from build123d import *

# Parameters (mm, degrees)
BOSS_EXTRUDE1_DEPTH = 4
CUT_EXTRUDE1_REACH  = 6
SKETCH2_R           = 11.5
SKETCH2_R_2         = 1.6
CUT_EXTRUDE2_REACH  = 6
SKETCH4_R           = 1.5
SKETCH5_W           = 10
SKETCH5_H           = 30
BOSS_EXTRUDE2_DEPTH = 12
FILLET1_R           = 1.5
CUT_EXTRUDE3_REACH  = 6
SKETCH6_R           = 4


with BuildPart() as part:
    # Sketch1 → Boss-Extrude1 (new body)
    with BuildSketch(Plane.XZ.offset(-57.396189287)):
        with BuildLine():
            Line((117.077991716, 202.076411562), (117.077991716, 81.069101486))
            add(Edge.make_bspline(
                [(111.081646754, 75.072756524), (117.077991716, 75.072756524), (117.077991716, 81.069101486)],
                knots=[5.498396131, 5.498396131, 5.498396131, 7.067974483, 7.067974483, 7.067974483], degree=2, weights=[1, 0.707537269, 1]))
            Line((111.081646754, 75.072756524), (4.474336679, 75.072756524))
            add(Edge.make_bspline(
                [(-1.522008284, 81.069101486), (-1.522008284, 75.072756524), (4.474336679, 75.072756524)],
                knots=[5.498396131, 5.498396131, 5.498396131, 7.067974483, 7.067974483, 7.067974483], degree=2, weights=[1, 0.707537269, 1]))
            Line((-1.522008284, 81.069101486), (-1.522008284, 202.076411562))
            add(Edge.make_bspline(
                [(4.474336679, 208.072756524), (-1.522008284, 208.072756524), (-1.522008284, 202.076411562)],
                knots=[5.498396131, 5.498396131, 5.498396131, 7.067974483, 7.067974483, 7.067974483], degree=2, weights=[1, 0.707537269, 1]))
            Line((4.474336679, 208.072756524), (111.081646754, 208.072756524))
            add(Edge.make_bspline(
                [(117.077991716, 202.076411562), (117.077991716, 208.072756524), (111.081646754, 208.072756524)],
                knots=[5.498396131, 5.498396131, 5.498396131, 7.067974483, 7.067974483, 7.067974483], degree=2, weights=[1, 0.707537269, 1]))
        make_face()
    extrude(amount=BOSS_EXTRUDE1_DEPTH)

    # Sketch2 → Cut-Extrude1 (cut, up to next)
    with BuildSketch(Plane.XZ.offset(-53.396189287), mode=Mode.PRIVATE) as cut_extrude1_sk1:
        with Locations((57.631208462, 183.071537466)):
            Circle(SKETCH2_R)
    cut_extrude1_tool1 = extrude(cut_extrude1_sk1.sketch, amount=-CUT_EXTRUDE1_REACH, mode=Mode.PRIVATE) & part.part
    add(cut_extrude1_tool1.solids().sort_by_distance((57.631208, 53.396189, 183.071537))[0], mode=Mode.SUBTRACT)
    # Sketch2 → Cut-Extrude1 (cut, up to next)
    with BuildSketch(Plane.XZ.offset(-53.396189287), mode=Mode.PRIVATE) as cut_extrude1_sk2:
        with Locations((73.131208462, 198.571537436)):
            Circle(SKETCH2_R_2)
    cut_extrude1_tool2 = extrude(cut_extrude1_sk2.sketch, amount=-CUT_EXTRUDE1_REACH, mode=Mode.PRIVATE) & part.part
    add(cut_extrude1_tool2.solids().sort_by_distance((73.131208, 53.396189, 198.571537))[0], mode=Mode.SUBTRACT)
    # Sketch2 → Cut-Extrude1 (cut, up to next)
    with BuildSketch(Plane.XZ.offset(-53.396189287), mode=Mode.PRIVATE) as cut_extrude1_sk3:
        with Locations((42.131208462, 198.571537436)):
            Circle(SKETCH2_R_2)
    cut_extrude1_tool3 = extrude(cut_extrude1_sk3.sketch, amount=-CUT_EXTRUDE1_REACH, mode=Mode.PRIVATE) & part.part
    add(cut_extrude1_tool3.solids().sort_by_distance((42.131208, 53.396189, 198.571537))[0], mode=Mode.SUBTRACT)
    # Sketch2 → Cut-Extrude1 (cut, up to next)
    with BuildSketch(Plane.XZ.offset(-53.396189287), mode=Mode.PRIVATE) as cut_extrude1_sk4:
        with Locations((42.131208462, 167.571537436)):
            Circle(SKETCH2_R_2)
    cut_extrude1_tool4 = extrude(cut_extrude1_sk4.sketch, amount=-CUT_EXTRUDE1_REACH, mode=Mode.PRIVATE) & part.part
    add(cut_extrude1_tool4.solids().sort_by_distance((42.131208, 53.396189, 167.571537))[0], mode=Mode.SUBTRACT)
    # Sketch2 → Cut-Extrude1 (cut, up to next)
    with BuildSketch(Plane.XZ.offset(-53.396189287), mode=Mode.PRIVATE) as cut_extrude1_sk5:
        with Locations((73.131208462, 167.571537436)):
            Circle(SKETCH2_R_2)
    cut_extrude1_tool5 = extrude(cut_extrude1_sk5.sketch, amount=-CUT_EXTRUDE1_REACH, mode=Mode.PRIVATE) & part.part
    add(cut_extrude1_tool5.solids().sort_by_distance((73.131208, 53.396189, 167.571537))[0], mode=Mode.SUBTRACT)

    # Sketch4 → Cut-Extrude2 (cut, up to next)
    with BuildSketch(Plane.XZ.offset(-53.396189287), mode=Mode.PRIVATE) as cut_extrude2_sk1:
        with Locations((8.994115753, 197.556632488)):
            Circle(SKETCH4_R)
    cut_extrude2_tool1 = extrude(cut_extrude2_sk1.sketch, amount=-CUT_EXTRUDE2_REACH, mode=Mode.PRIVATE) & part.part
    add(cut_extrude2_tool1.solids().sort_by_distance((8.994116, 53.396189, 197.556632))[0], mode=Mode.SUBTRACT)
    # Sketch4 → Cut-Extrude2 (cut, up to next)
    with BuildSketch(Plane.XZ.offset(-53.396189287), mode=Mode.PRIVATE) as cut_extrude2_sk2:
        with Locations((106.56186768, 197.556632488)):
            Circle(SKETCH4_R)
    cut_extrude2_tool2 = extrude(cut_extrude2_sk2.sketch, amount=-CUT_EXTRUDE2_REACH, mode=Mode.PRIVATE) & part.part
    add(cut_extrude2_tool2.solids().sort_by_distance((106.561868, 53.396189, 197.556632))[0], mode=Mode.SUBTRACT)
    # Sketch4 → Cut-Extrude2 (cut, up to next)
    with BuildSketch(Plane.XZ.offset(-53.396189287), mode=Mode.PRIVATE) as cut_extrude2_sk3:
        with Locations((8.994115753, 85.588880561)):
            Circle(SKETCH4_R)
    cut_extrude2_tool3 = extrude(cut_extrude2_sk3.sketch, amount=-CUT_EXTRUDE2_REACH, mode=Mode.PRIVATE) & part.part
    add(cut_extrude2_tool3.solids().sort_by_distance((8.994116, 53.396189, 85.588881))[0], mode=Mode.SUBTRACT)
    # Sketch4 → Cut-Extrude2 (cut, up to next)
    with BuildSketch(Plane.XZ.offset(-53.396189287), mode=Mode.PRIVATE) as cut_extrude2_sk4:
        with Locations((106.56186768, 85.588880561)):
            Circle(SKETCH4_R)
    cut_extrude2_tool4 = extrude(cut_extrude2_sk4.sketch, amount=-CUT_EXTRUDE2_REACH, mode=Mode.PRIVATE) & part.part
    add(cut_extrude2_tool4.solids().sort_by_distance((106.561868, 53.396189, 85.588881))[0], mode=Mode.SUBTRACT)

    # Sketch5 → Boss-Extrude2 (add)
    with BuildSketch(Plane.XZ.offset(-53.396189287)):
        with Locations((57.477991716, 148.072756524)):
            Rectangle(SKETCH5_W, SKETCH5_H)
    extrude(amount=BOSS_EXTRUDE2_DEPTH)

    # Fillet1
    fillet1_edges = [part.edges().sort_by_distance(p)[0] for p in [
        (52.477991716, 53.396189287, 148.072756524),
        (52.477991716, 47.396189287, 163.072756524),
        (57.477991716, 53.396189287, 133.072756524),
        (52.477991716, 47.396189287, 133.072756524),
        (62.477991716, 53.396189287, 148.072756524),
        (62.477991716, 47.396189287, 133.072756524),
        (57.477991716, 53.396189287, 163.072756524),
        (62.477991716, 47.396189287, 163.072756524),
    ]]
    fillet(fillet1_edges, radius=FILLET1_R)

    # Sketch6 → Cut-Extrude3 (cut, up to next)
    with BuildSketch(Plane.XZ.offset(-53.396189287), mode=Mode.PRIVATE) as cut_extrude3_sk1:
        with Locations((38.477991716, 158.072756524)):
            Circle(SKETCH6_R)
    cut_extrude3_tool1 = extrude(cut_extrude3_sk1.sketch, amount=-CUT_EXTRUDE3_REACH, mode=Mode.PRIVATE) & part.part
    add(cut_extrude3_tool1.solids().sort_by_distance((38.477992, 53.396189, 158.072757))[0], mode=Mode.SUBTRACT)


solid = part.part
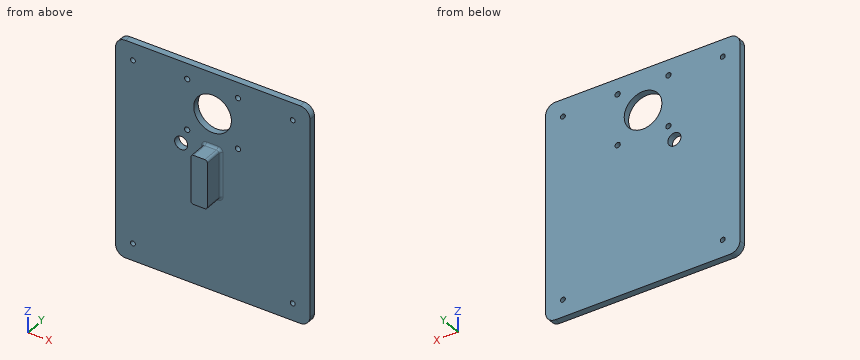
Model file for the job. Use its own axes, mm. Give positions to 0.01 mm unless a question says otherwise; leave off trailing zeros. Loops run counter-clockwise (first coordinate to the right, second up) from the corner with the lowest first, then second, coordinate; pieces in that order, holes last.
1) Saw through at C-C (x = 58). Write the cut outline in (y, z).
2) Wall check: line 1 (Y direction, x = 71, z = 169); line 2 (X direction, y = 49, z = 161.5); line 3 (X direction, y = 55, z = 84.5). Give the ranges that are in metal, low to high.
3) Flat gauge pins, fed straight in: pin 1 Ø5 at (x, z) = (106.56, 197.56) entering from +Y; pin 2 Ø7.5 at (x, y) = (56, 46) entering from -Z; pin 3 Ø5 at (x, z) = (38.48, 158.07) entering from -Y; pin 4 Ø2 at (x, y) = (58.5, 45) entering from +Z. Where does each tip first touch, or does it go through?
4) Saw through at A-A (y = 45). Write the cut outline in (x, z).
5) Saw through at D-D (x = 83). Write the cut outline in (y, z).
6) Saw through at B-B (z = 186). Write the cut outline in (x, y), plus the area to 3 significant figures.
Answer block:
1. outline: (41.4, 133.07) - (51.9, 133.07) arc R1.5 cw to (53.4, 131.57) - (53.4, 75.07) - (57.4, 75.07) - (57.4, 171.58) - (53.4, 171.58) - (53.4, 164.57) arc R1.5 cw to (51.9, 163.07) - (41.4, 163.07) - close; (53.4, 194.57) - (57.4, 194.57) - (57.4, 208.07) - (53.4, 208.07) - close
2. line 1: y = 53.4 to 57.4
2. line 2: x = 52.48 to 62.48
2. line 3: x = -1.52 to 7.96, 10.03 to 105.53, 107.59 to 117.08
3. pin 1: stops at y = 57.4
3. pin 2: stops at z = 133.07
3. pin 3: passes through
3. pin 4: stops at z = 163.07
4. outline: (52.48, 134.57) arc R1.5 ccw to (53.98, 133.07) - (60.98, 133.07) arc R1.5 ccw to (62.48, 134.57) - (62.48, 161.57) arc R1.5 ccw to (60.98, 163.07) - (53.98, 163.07) arc R1.5 ccw to (52.48, 161.57) - close
5. outline: (53.4, 75.07) - (57.4, 75.07) - (57.4, 208.07) - (53.4, 208.07) - close
6. outline: (-1.52, 53.4) - (46.51, 53.4) - (46.51, 57.4) - (-1.52, 57.4) - close; (68.75, 53.4) - (117.08, 53.4) - (117.08, 57.4) - (68.75, 57.4) - close
6. area: 385 mm2
